The listing builds one solid part. Answer for the finished solid, in the listing's coordinates (mm). Face numbers are marked on the shaded views. A direction names the side the tool comes from. Coordinates: 2 decimals unless noted, no trailing zeros. Order: outer loops, then holes, each group sorted by start corner. A loop starts at its lowest first (then second) coordinate and runs counter-clockwise, first axis right, second up. Notation, with made-up numbers: (54.5, 65.25) -> (63.5, 65.25) arc R25 cw to (63.5, 86.25) -> close; hole circle Ø5 at (-8, 4). An arc over 180 degrees is marked (long way). One line per question, with ' | ' between items.
from build123d import *

# Parameters (mm, degrees)
SKETCH1_W           = 20
SKETCH1_H           = 30
BOSS_EXTRUDE1_DEPTH = 7
SKETCH2_W           = 30
SKETCH2_H           = 5
CUT_EXTRUDE1_DEPTH  = 2
SKETCH3_W           = 30
SKETCH3_H           = 5
CUT_EXTRUDE2_DEPTH  = 2
SKETCH4_R           = 3.85
BOSS_EXTRUDE2_DEPTH = 7.5


with BuildPart() as part:
    # Sketch1 → Boss-Extrude1 (new body)
    with BuildSketch(Plane(origin=(0, 0, 0), x_dir=(1, 0, 0), z_dir=(0, 1, 0))):
        Rectangle(SKETCH1_W, SKETCH1_H)
    extrude(amount=BOSS_EXTRUDE1_DEPTH)

    # Sketch2 → Cut-Extrude1 (cut)
    with BuildSketch(Plane(origin=(10, 0, 0), x_dir=(0, 0, -1), z_dir=(1, 0, 0))):
        with Locations((0, 3.5)):
            Rectangle(SKETCH2_W, SKETCH2_H)
    extrude(amount=-CUT_EXTRUDE1_DEPTH, mode=Mode.SUBTRACT)

    # Sketch3 → Cut-Extrude2 (cut)
    with BuildSketch(Plane.ZY.offset(10)):
        with Locations((0, 3.5)):
            Rectangle(SKETCH3_W, SKETCH3_H)
    extrude(amount=-CUT_EXTRUDE2_DEPTH, mode=Mode.SUBTRACT)

    # Sketch4 → Boss-Extrude2 (add)
    with BuildSketch(Plane(origin=(0, 7, 0), x_dir=(1, 0, 0), z_dir=(0, 1, 0))):
        Circle(SKETCH4_R)
    extrude(amount=BOSS_EXTRUDE2_DEPTH)


solid = part.part
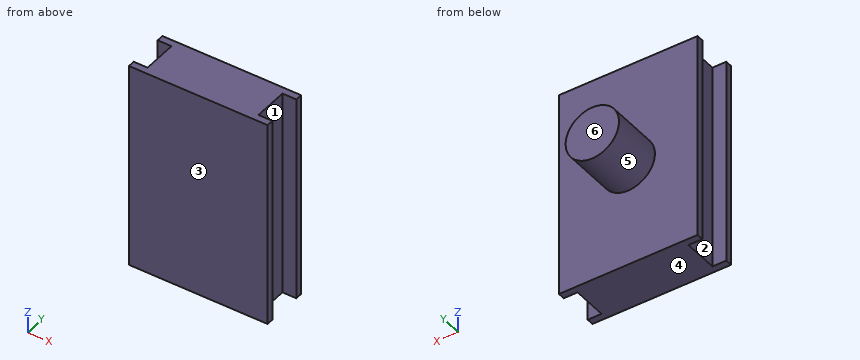
Item 1: Section D-D, the plane y = 11.5 is taken. Give the vertices of the cut face in (x, z), plus the area to 3 significant figures.
Computed values:
outline: circle Ø7.7 at (0, 0) | area: 46.6 mm^2
Item 2: Section A-A, the plane x = 8.75 is taken. Give the vertices of the cut face in (y, z), plus the area to 3 significant figures.
Computed values:
outline: (0, -15) -> (1, -15) -> (1, 15) -> (0, 15) -> close; (6, -15) -> (7, -15) -> (7, 15) -> (6, 15) -> close | area: 60.0 mm^2
Item 3: Find the intervals of material crossed by L1, parallel to Y at x = -8.5, z = -12.25; L2, parallel to Y at x = 1, z = -5; L3, parallel to X at y = 1.5, z = 0, in increasing order.
Computed values:
L1: y = 0 to 1, 6 to 7 | L2: y = 0 to 7 | L3: x = -8 to 8
Item 4: Section B-B, the plane z = 0 is taken. Give the vertices of the cut face in (x, y).
Computed values:
outline: (-10, 0) -> (10, 0) -> (10, 1) -> (8, 1) -> (8, 6) -> (10, 6) -> (10, 7) -> (3.85, 7) -> (3.85, 14.5) -> (-3.85, 14.5) -> (-3.85, 7) -> (-10, 7) -> (-10, 6) -> (-8, 6) -> (-8, 1) -> (-10, 1) -> close
Item 5: Determine the mould class of the marked faces 1, 2, 3 and 4 for opening direction Y: pulls with the +Y half, pulls with the -Y half, needs draft (parallel to the pull), parting line crosses it, or undercut.
Computed values:
face 1: undercut | face 2: undercut | face 3: pulls with the -Y half | face 4: needs draft
Item 6: For the marked faces 5 and 6, determine the directions among +Z, -Z, +X, -X, +Y, -Y from which every point of the face is accessible in a straight line to the end or side of a thin tool.
Computed values:
face 5: +Y | face 6: +Z, -Z, +X, -X, +Y
Item 7: Each of these flat-tipped pins is pushed along its axis until it touches: pin 1 Ø1.6 at (x, z) = (9, 3) entering from +Y; pin 2 Ø3 at (y, z) = (12.5, -1) entering from +X; pin 3 Ø5 at (y, z) = (12, -1.5) entering from -X. Where does it stop, or does it pass through?
Computed values:
pin 1: stops at y = 7 | pin 2: stops at x = 3.85 | pin 3: stops at x = -3.85
Item 8: Section C-C, the plane x = 0 is taken. Give the vertices of the cut face in (y, z).
Computed values:
outline: (0, -15) -> (7, -15) -> (7, -3.85) -> (14.5, -3.85) -> (14.5, 3.85) -> (7, 3.85) -> (7, 15) -> (0, 15) -> close
